Here's how the part is built. I have some questions about the finished solid (model axes, mm). Face numbers are marked on the shaded views. A direction names the side the tool comes from. Give positions to 0.01 mm unless a question says otherwise; leave off trailing zeros. Order: outer loops, then holes, each group sorted by start corner. A loop starts at its lowest first (then second) coordinate and runs counter-clockwise, first axis right, second up.
from build123d import *

# Parameters (mm, degrees)
SKETCH_1_R          = 6.4
EXTRUDE_1_DEPTH     = 5.4
SKETCH_2_R          = 3.985
EXTRUDE_2_DEPTH     = 30
SKETCH_3_R          = 3
EXTRUDE_3_DEPTH     = 11.25
CHAMFER_1_SIZE      = 1
CHAMFER_1_SIZE2     = 0.839099631
CUT_EXTRUDE_1_DEPTH = 3


with BuildPart() as part:
    # 草图1 → 凸台-拉伸1 (new body)
    with BuildSketch(Plane(origin=(0, 0, 0), x_dir=(1, 0, 0), z_dir=(0, 1, 0))):
        with Locations(Location((0, 0, 0), (0, 0, 90))):
            Circle(SKETCH_1_R)
    extrude(amount=EXTRUDE_1_DEPTH)

    # 草图2 → 凸台-拉伸2 (add)
    with BuildSketch(Plane(origin=(0, 5.4, 0), x_dir=(1, 0, 0), z_dir=(0, 1, 0))):
        with Locations(Location((0, 0, 0), (0, 0, 270))):
            Circle(SKETCH_2_R)
    extrude(amount=EXTRUDE_2_DEPTH)

    # 草图3 → 凸台-拉伸3 (add)
    with BuildSketch(Plane(origin=(0, 35.4, 0), x_dir=(1, 0, 0), z_dir=(0, 1, 0))):
        with Locations(Location((0, 0, 0), (0, 0, 90))):
            Circle(SKETCH_3_R)
    extrude(amount=EXTRUDE_3_DEPTH)

    # 倒角1
    chamfer_1_edges = [part.edges().sort_by_distance(p)[0] for p in [
        (0, 0, 6.4),
    ]]
    chamfer_1_side = [part.faces().sort_by_distance(p)[0] for p in [
        (0, 0, 0),
    ]]
    chamfer(chamfer_1_edges, length=CHAMFER_1_SIZE, length2=CHAMFER_1_SIZE2, reference=chamfer_1_side[0])

    # 草图4 → 切除-拉伸1 (cut)
    with BuildSketch(Plane.XZ):
        Polygon((0, 2.309401077), (-2, 1.154700538), (-2, -1.154700538), (0, -2.309401077), (2, -1.154700538), (2, 1.154700538), align=None)
    extrude(amount=-CUT_EXTRUDE_1_DEPTH, mode=Mode.SUBTRACT)


solid = part.part
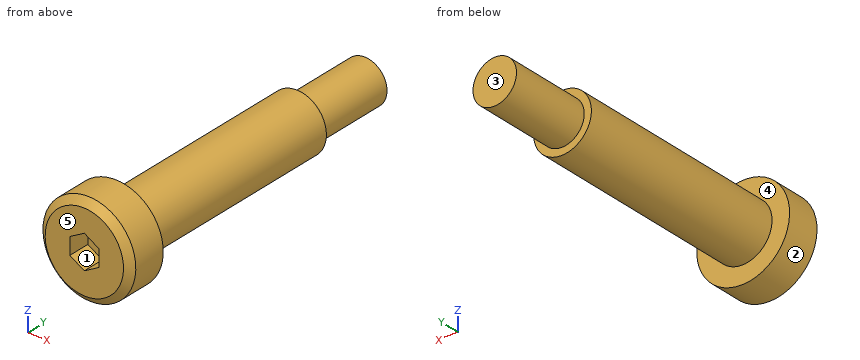
Q1. If we section it at A-A on z = 0: List the corners of the cut face in (x, y) for me (3 decimals).
Filled sheet:
outline: (-6.4, 0.839) - (-5.4, 0) - (-2, 0) - (-2, 3) - (2, 3) - (2, 0) - (5.4, 0) - (6.4, 0.839) - (6.4, 5.4) - (3.985, 5.4) - (3.985, 35.4) - (3, 35.4) - (3, 46.65) - (-3, 46.65) - (-3, 35.4) - (-3.985, 35.4) - (-3.985, 5.4) - (-6.4, 5.4) - close
Q2. I need wall thicknesses on L1, parallel to Y at x = 1.75, z = -4.5; L2, parallel to Y at x = 2.25, z = -2.5; L3, parallel to X at y = 26, z = 1. Which ranges of each line are inside material? Lowest first, please.
Filled sheet:
L1: y = 0 to 5.4
L2: y = 0 to 35.4
L3: x = -3.86 to 3.86
Q3. I'm going to push flat-ended pins straight in: P1, Ø2, axis at x = 0.5, y = 19, coming from the +Z side (3 decimals); P2, Ø4, axis at x = 5, y = 23, coming from the +Z side; P3, Ø5, axis at x = -5, z = -4, coming from the +Y side. Where does each tip first touch, or does it pass through?
Filled sheet:
P1: stops at z = 3.985
P2: stops at z = 2.62
P3: stops at y = 35.4
Q4. Thinking about a two-plate mould opening in Z: for the marked faces 1, 2 and 3, which applies, released by +Z, released by -Z, zero draft, split by the parting line, or undercut?
Filled sheet:
face 1: undercut
face 2: split by the parting line
face 3: zero draft
Q5. For the marked faces 4 and 5, which set-ups out of +Z, -Z, +X, -X, +Y, -Y let a thin tool reach every point of the face, with its end or its side?
Filled sheet:
face 4: +Y
face 5: +Z, -Z, +X, -X, -Y
Q6. If we section it at B-B on y = 32: List the corners of the cut face in (x, z) for me (3 decimals).
Filled sheet:
outline: circle Ø7.97 at (0, 0)
